Solid Edge part; units mm, degrees
sketch "Sketch1" plane through (0, 0, 0) normal (0, 0, 1) x (1, 0, 0)
  line L0 (120, 40) -> (0, 40)
  line L1 (0, 40) -> (0, 0)
  line L2 (0, 0) -> (120, 0)
  line L3 (120, 0) -> (120, 40)
extrude "Protrusion1" add sketch "Sketch1" along normal blind 5
sketch "Sketch2" plane through (60, 20, 5) normal (0, 0, 1) x (1, 0, 0)
  line L0 (55, -20) -> (55, 20)
  line L1 (55, 20) -> (60, 20)
  line L2 (60, 20) -> (60, -20)
  line L3 (60, -20) -> (55, -20)
  line L4 (-55, 20) -> (-55, -20)
  line L5 (-55, -20) -> (-60, -20)
  line L6 (-60, -20) -> (-60, 20)
  line L7 (-60, 20) -> (-55, 20)
extrude "Extrusionsausprägung_2" add sketch "Sketch2" along normal blind 60
hole "Bohrung_1" at (120, 20, 45) direction (-1, 0, 0) diameter 10 end through all
hole "Hole_2" at (20, 10, 5) direction (0, 0, -1) diameter 4.2 end up to next start chamfer 0.6 start chamfer angle 45
hole "Hole1" at (20, 30, 5) direction (0, 0, -1) diameter 4.2 end up to next start chamfer 0.6 start chamfer angle 45
hole "Hole2" at (100, 30, 5) direction (0, 0, -1) diameter 4.2 end up to next start chamfer 0.6 start chamfer angle 45
hole "Hole3" at (100, 10, 5) direction (0, 0, -1) diameter 4.2 end up to next start chamfer 0.6 start chamfer angle 45
hole "Hole4" at (120, 9, 56) direction (-1, 0, 0) diameter 4.2 end up to next
hole "Hole5" at (120, 9, 34) direction (-1, 0, 0) diameter 4.2 end up to next
hole "Hole6" at (120, 31, 34) direction (-1, 0, 0) diameter 4.2 end up to next
hole "Hole7" at (120, 31, 56) direction (-1, 0, 0) diameter 4.2 end up to next
Geometry check sheet. Reference: the model listing, model coordinates, mm. A direction names the side the tool comes from. Give positions to 0.01 mm unless a question says otherwise; leave off trailing zeros. Loops run counter-clockwise (first coordinate to the right, second up) from the corner with the lowest first, then second, coordinate; pieces in that order, holes last. Notation, with made-up numbers: M 51,64.5 L 93,64.5 A29 ccw 93,103.5 Z; hole C 46.5,-3 d10. An arc over 180 degrees is marked long. Write each question's results on one line, items separated by ' | '.
1) Release check for a two-part mould opening along X. For faces 4 (the face through (0, 20, 32)), 5 (the face through (117.535, 29.722, 35.666)), 6 (the face through (59, 20, 5)), 7 (the face through (120, 20, 32)) record: +X half, -X half, draft (parallel to the pull), parting line (faces both ways), or undercut.
Answers follow:
face 4: -X half | face 5: draft | face 6: undercut | face 7: +X half
2) Tool access check on faces 1 (the face through (115, 20, 35)), 2 (the face through (117.535, 29.137, 55.031)), 3 (the face through (118, 17, 49)). Record the directions out of +Z, -Z, +X, -X, +Y, -Y that give a thin tool (end or side, any length) a straight path to the whole face; none if there is none.
Answers follow:
face 1: +Z, +Y, -Y | face 2: +X | face 3: +X, -X
3) Section check A-A, the plane z = 23. Record the boundary of the cut face in (x, y).
Answers follow:
outline: M 0,0 L 5,0 L 5,40 L 0,40 Z; M 115,0 L 120,0 L 120,40 L 115,40 Z
4) Section check B-B, the plane x = 100. Record the boundary of the cut face in (y, z).
Answers follow:
outline: M 0,0 L 7.9,0 L 7.9,4.4 L 7.3,5 L 0,5 Z; M 12.1,0 L 27.9,0 L 27.9,4.4 L 27.3,5 L 12.7,5 L 12.1,4.4 Z; M 32.1,0 L 40,0 L 40,5 L 32.7,5 L 32.1,4.4 Z
5) Section check C-C, the plane y = 20. Record the boundary of the cut face in (x, z), plus the area to 3 significant figures.
Answers follow:
outline: M 0,0 L 120,0 L 120,40 L 115,40 L 115,5 L 5,5 L 5,40 L 0,40 Z; M 0,50 L 5,50 L 5,65 L 0,65 Z; M 115,50 L 120,50 L 120,65 L 115,65 Z | area: 1,100 mm2
6) Gauge pin test, flat ends, axial feed: pin 1 (12 mm diameter, centred on x = 37.5, y = 13, fed in from +Z); pin 2 (5 mm diameter, centred on x = 20, y = 10, fed in from +Z). Record the tip position at first contact, or that the pin passes through.
Answers follow:
pin 1: z = 5 | pin 2: z = 4.8
7) Thickness scan on line 1 (Y direction, x = 118, z = 34); line 2 (Z direction, x = 116.6, y = 31); line 3 (Y direction, x = 100, z = 1). Record the ranges inside material, lowest first.
Answers follow:
line 1: 0 to 6.9, 11.1 to 28.9, 33.1 to 40 | line 2: 0 to 31.9, 36.1 to 53.9, 58.1 to 65 | line 3: 0 to 7.9, 12.1 to 27.9, 32.1 to 40
8) Section check D-D, the plane z = 45. Record the boundary of the cut face in (x, y).
Answers follow:
outline: M 0,0 L 5,0 L 5,15 L 0,15 Z; M 0,25 L 5,25 L 5,40 L 0,40 Z; M 115,0 L 120,0 L 120,15 L 115,15 Z; M 115,25 L 120,25 L 120,40 L 115,40 Z
